Could you check a few things on this drawing? It's one solid part, dimensions in mm from its lowest x, y, z. Coordinates: 2 decimals unless noted, no trailing zeros. Order: outer loops, then holes, each group sorted by start corner. A loop starts at its lowest first (then second) coordinate and runs counter-clockwise, first axis right, second up.
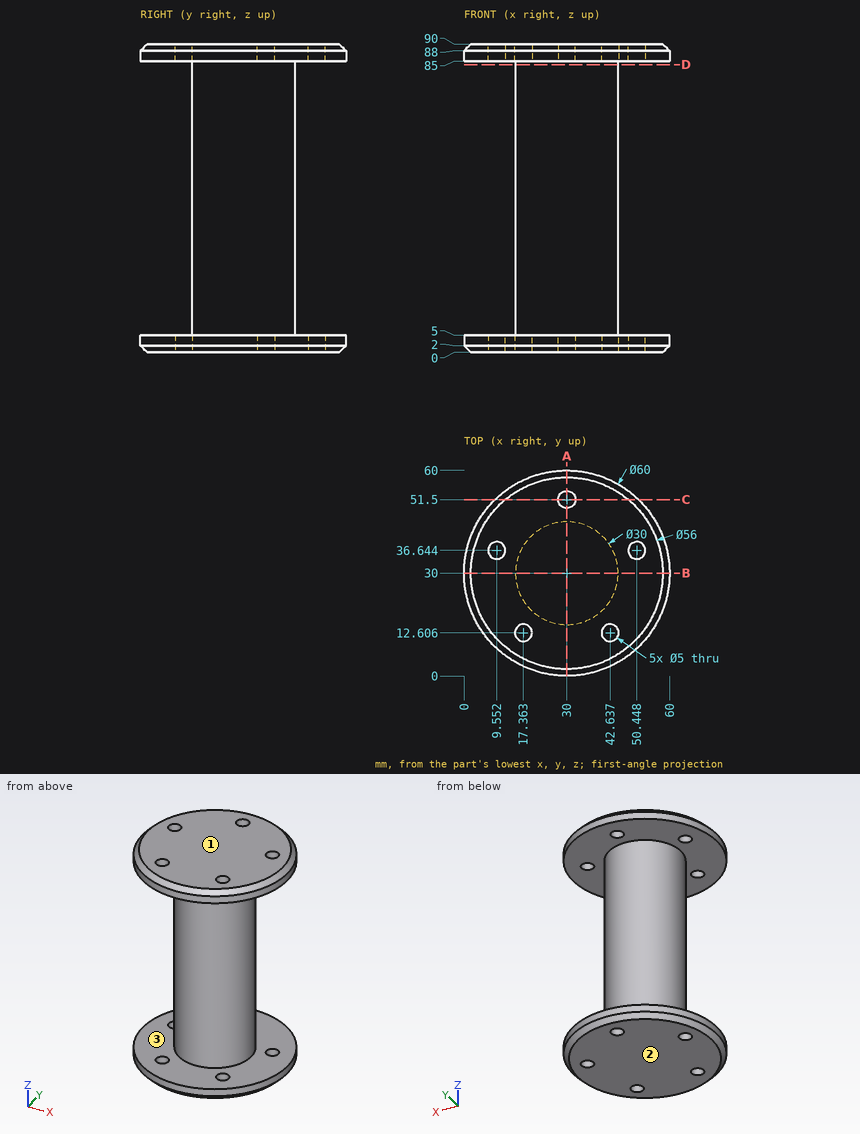
1. I'm going to push flat-ended pins straight in: pin 1 (5 mm diameter, centred on x = 25.5, z = 79, fed in from -Y); pin 2 (6 mm diameter, centred on x = 32, z = 18.5, fed in from -Y); pin 3 (1.5 mm diameter, centred on y = 44.5, z = 55.5, fed in from +X) (1 decimal). Where does each tip first touch, or does it pass through?
Completed:
pin 1: stops at y = 15.13
pin 2: stops at y = 15
pin 3: stops at x = 36
2. Imagine slicing it at C-C on y = 51.5. Give the number of separate pieces and of enclosed holes in the cut face, then the cut area to 3 significant figures.
Completed:
separate pieces: 4
enclosed holes: 0
area: 357 mm2
3. Imagine slicing it at B-B on y = 30. Please give me the cut outline in (x, z).
Completed:
outline: (0, 2) - (2, 0) - (58, 0) - (60, 2) - (60, 5) - (45, 5) - (45, 85) - (60, 85) - (60, 88) - (58, 90) - (2, 90) - (0, 88) - (0, 85) - (15, 85) - (15, 5) - (0, 5) - close
4. Imagine slicing it at A-A on x = 30. Please give me the cut outline in (y, z).
Completed:
outline: (0, 2) - (2, 0) - (49, 0) - (49, 5) - (45, 5) - (45, 85) - (49, 85) - (49, 90) - (2, 90) - (0, 88) - (0, 85) - (15, 85) - (15, 5) - (0, 5) - close; (54, 0) - (58, 0) - (60, 2) - (60, 5) - (54, 5) - close; (54, 85) - (60, 85) - (60, 88) - (58, 90) - (54, 90) - close
5. Imagine slicing it at D-D on z = 84. Please give me the cut outline in (x, y), then the cut area to 3 significant figures.
Completed:
outline: circle Ø30 at (30, 30)
area: 707 mm2
6. Thinking about a two-plate mould opening in Z: for the marked faces 1, 2 and 3, which applies, pulls with the +Z half, pulls with the -Z half, needs draft (parallel to the pull), parting line crosses it, or undercut?
Completed:
face 1: pulls with the +Z half
face 2: pulls with the -Z half
face 3: undercut
7. Please list where these lines run through material, in increasing order: probe 1 along Z at (x, y) = (6, 34.5); probe 2 along Z at (x, y) = (47, 54.5); probe 3 along Y at (x, z) = (30, 2.65).
Completed:
probe 1: z = 0 to 5, 85 to 90
probe 2: z = 1.82 to 5, 85 to 88.18
probe 3: y = 0 to 49, 54 to 60
